The listing builds one solid part. Answer for the finished solid, in the listing's coordinates (mm). Face numbers are marked on the shaded views. A direction names the side the tool comes from. Round coordinates to 2 decimals unless told otherwise and drop trailing zeros. Write each loop counter-clockwise with the first axis right and the second up, starting at its lowest first coordinate (ties: lowest second). Pieces come first, ordered by that corner, then holes. Notation, with made-up numbers: (-32.75, -1.5) - (-20.75, -1.5) arc R18 cw to (-20.75, 22.5) - close; hole circle Ø3 at (23.25, 52.5). An arc over 180 degrees is marked (long way). Answer in a Markdown table with one row per item.
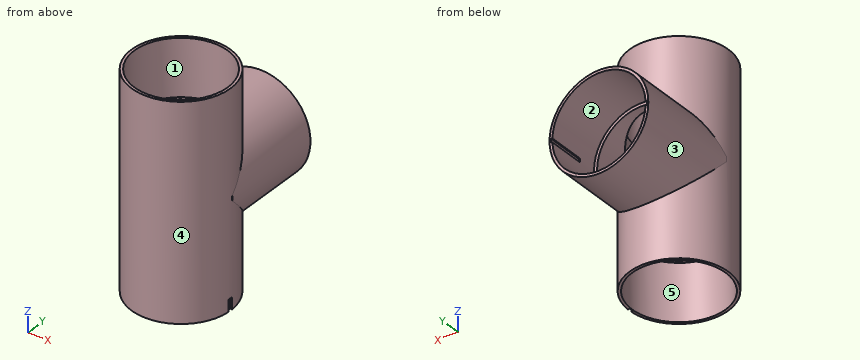
Autodesk Inventor part; units mm, degrees
ref_plane "Work Plane5" through (0, 33.45, 143.5) normal (0, 1, 0) x (-1, 0, 0)
ref_plane "Work Plane6" through (32, 0, 0) normal (1, 0, 0) x (0, 1, 0)
ref_plane "XZ Plane" through (0, 0, 0) normal (0, 1, 0) x (-1, 0, 0)
sketch "Sketch1" plane through (0, 0, 0) normal (0, 0, 1) x (1, 0, 0)
  circle A0 centre (0, 0) radius 33.45
  dimension "d0" = 66.9
extrude "mainBody" add sketch "Sketch1" along normal blind 143.5
sketch "Sketch10" plane through (0, 0, 143.5) normal (0, 0, 1) x (1, 0, 0)
  circle A0 centre (0, 0) radius 30.1625
  circle A1 centre (0, 0) radius 33.45
  point P0 (0, 33.45)
ref_plane "Work Plane5" through (0, 33.45, 143.5) normal (0, 1, 0) x (-1, 0, 0)
sketch "Sketch11" plane through (0, 33.45, 143.5) normal (0, 1, 0) x (-1, 0, 0)
  circle A0 centre (0, -71.75) radius 33.45
  line L0 (33.45, 0) -> (-33.45, 0)
  point P0 (0, -143.5)
  dimension "d29" = 71.75
  dimension "d30" = 66.9
extrude "TBody" add sketch "Sketch11" along normal blind 40 and the other way blind 31.75
sketch "Sketch12" plane through (0, 73.45, 71.75) normal (0, 1, 0) x (1, 0, 0)
  circle A0 centre (0, 0) radius 33.45
  circle A1 centre (0, 0) radius 31.6
  point P0 (0, 71.75)
  dimension "d35" = 63.2
extrude "TSocket" cut sketch "Sketch12" against normal blind 38.3 contours A1
sketch "Sketch13" plane through (0, 35.15, 71.75) normal (0, 1, 0) x (1, 0, 0)
  circle A0 centre (0, 0) radius 31.6
  circle A1 centre (0, 0) radius 29.5
  point P0 (0, 71.75)
  dimension "d39" = 59
extrude "TTube" cut sketch "Sketch13" against normal blind 38.1 contours A1
sketch "Sketch14" plane through (0, 0, 143.5) normal (0, 0, 1) x (1, 0, 0)
  circle A0 centre (0, 0) radius 33.45
  circle A1 centre (0, 0) radius 29.5
  dimension "d43" = 59
extrude "mainTube" cut sketch "Sketch14" against normal blind 177.8 contours A1
sketch "Sketch15" plane through (0, 0, 143.5) normal (0, 0, 1) x (1, 0, 0)
  circle A0 centre (0, 0) radius 29.5
  circle A1 centre (0, 0) radius 33.45
  circle A2 centre (0, 0) radius 31.6
  dimension "d47" = 63.2
extrude "mainSocket1" cut sketch "Sketch15" against normal blind 38.3 contours A2
sketch "Sketch16" plane through (0, 0, 0) normal (0, 0, -1) x (-1, 0, 0)
  circle A0 centre (0, 0) radius 29.5
  circle A1 centre (0, 0) radius 33.45
  circle A2 centre (0, 0) radius 31.6
  dimension "d51" = 63.2
extrude "mainSocket2" cut sketch "Sketch16" against normal blind 38.3 contours A2
sketch "Sketch24" plane through (0, 73.45, 71.75) normal (0, 1, 0) x (1, 0, 0)
  circle A0 centre (0, 0) radius 31.6
  line L0 (-31.6, 0) -> (31.6, 0) construction
  line L1 (0, 31.6) -> (0, -31.6) construction
  line L2 (-32.3825, -1.27) -> (-28.3825, -1.27)
  line L3 (-28.3825, -1.27) -> (-28.3825, 1.27)
  line L4 (-28.3825, 1.27) -> (-32.3825, 1.27)
  line L5 (-32.3825, 1.27) -> (-32.3825, -1.27)
  line L6 (-32.3825, 0) -> (-28.3825, 0) construction
  line L7 (32.3825, -1.27) -> (28.3825, -1.27)
  line L8 (28.3825, -1.27) -> (28.3825, 1.27)
  line L9 (28.3825, 1.27) -> (32.3825, 1.27)
  line L10 (32.3825, 1.27) -> (32.3825, -1.27)
  line L11 (32.3825, 0) -> (28.3825, 0) construction
  point P0 (0, 71.75)
  dimension "d72" = 4
  dimension "d75" = 2.54
extrude "Extrusion20" cut sketch "Sketch24" against normal blind 25.4 contours A0 L7 L8 L9 | A0 L9 L10 L7 | L4 L3 L2 A0 | A0 L2 L5 L4
ref_plane "Work Plane6" through (32, 0, 0) normal (1, 0, 0) x (0, 1, 0)
sketch "Sketch27" plane through (32, 0, 0) normal (1, 0, 0) x (0, 1, 0)
  line L0 (-1.5232, -1.2223) -> (1.5232, -1.2223)
  line L1 (1.5232, -1.2223) -> (1.5232, 8.0295)
  line L2 (1.5232, 8.0295) -> (-1.5232, 8.0295)
  line L3 (-1.5232, 8.0295) -> (-1.5232, -1.2223)
  point P0 (0, 0)
extrude "Extrusion22" cut sketch "Sketch27" along normal blind 25.4
equation "\"d1\" = length"
equation "\"d29\" = 0.5 * length"
equation "\"length\" = 143.5"
properties part number "0pvc_T_2in" material "PVC-Piping"
(1) Section D-D (y = -14) is taken. Give the vertices of the cut face in (x, z).
Checked values:
| item | result |
|---|---|
| outline | (-30.38, 0) - (-28.33, 0) - (-28.33, 38.3) - (-25.97, 38.3) - (-25.97, 105.2) - (-28.33, 105.2) - (-28.33, 143.5) - (-30.38, 143.5) - close; (25.97, 38.3) - (28.33, 38.3) - (28.33, 0) - (30.38, 0) - (30.38, 143.5) - (28.33, 143.5) - (28.33, 105.2) - (25.97, 105.2) - close |
(2) Flat-ended cylindrical pins translate along their axes: pin 1 (5 mm diameter, centred on x = 11.5, z = 14.5, fed in from -Y); pin 2 (1 mm diameter, centred on x = -3.5, z = 98.5, fed in from -Y); pin 3 (12 mm diameter, centred on x = 5.5, y = 53.5, fed in from -Z). Find the tip coordinate at first contact, or state that the pin passes through.
Checked values:
| item | result |
|---|---|
| pin 1 | stops at y = -32.22 |
| pin 2 | stops at y = -33.32 |
| pin 3 | stops at z = 38.3 |
(3) Section A-A (x = 0) is taken. Give the vertices of the cut face in (y, z).
Checked values:
| item | result |
|---|---|
| outline | (-33.45, 0) - (-31.6, 0) - (-31.6, 38.3) - (-29.5, 38.3) - (-29.5, 105.2) - (-31.6, 105.2) - (-31.6, 143.5) - (-33.45, 143.5) - close; (29.5, 38.3) - (31.6, 38.3) - (31.6, 0) - (33.45, 0) - (33.45, 38.3) - (73.45, 38.3) - (73.45, 40.15) - (35.15, 40.15) - (35.15, 42.25) - (29.5, 42.25) - close; (29.5, 101.25) - (35.15, 101.25) - (35.15, 103.35) - (73.45, 103.35) - (73.45, 105.2) - (33.45, 105.2) - (33.45, 143.5) - (31.6, 143.5) - (31.6, 105.2) - (29.5, 105.2) - close |
(4) Section C-C (z = 112.5) is taken. Give the vertices of the cut face in (x, y).
Checked values:
| item | result |
|---|---|
| outline | circle Ø66.9 at (0, 0); hole circle Ø63.2 at (0, 0) |
(5) For a pull along Y with two mould halves and no side action, classify the marked faces 3, 4 and 5 as pulls with the +Y half, pulls with the -Y half, needs draft (parallel to the pull), parting line crosses it, or undercut.
Checked values:
| item | result |
|---|---|
| face 3 | needs draft |
| face 4 | parting line crosses it |
| face 5 | undercut |
(6) For the marked faces 1 and 2, determine the directions among +Z, -Z, +X, -X, +Y, -Y from which every point of the face is accessible in a straight line to the end or side of a thin tool.
Checked values:
| item | result |
|---|---|
| face 1 | +Z |
| face 2 | +Y |
(7) Find the intervals of material crossed by line 1 (X direction, y = 10, z = 71); line 2 (Y direction, x = 0, z = 10.5); line 3 (X direction, y = 60, z = 71.75), in increasing order.
Checked values:
| item | result |
|---|---|
| line 1 | x = -33.44 to -29.49, 29.49 to 33.44 |
| line 2 | y = -33.45 to -31.6, 31.6 to 33.45 |
| line 3 | x = -33.45 to -32.38, 32.38 to 33.45 |
